Geometry check sheet. Reference: the model listing, model coordinates, mm. Round coordinates to 2 decimals unless told otherwise and drop trailing zeros. Write each loop counter-clockwise with the first axis right and the second up, starting at its lowest first coordinate (ties: lowest second). Pieces come first, ordered by that corner, then holes. Notation, with made-up numbers: M 37,11 L 53,11 A17 cw 53,25 Z; hole C 31,42.5 d4. An arc over 180 degrees is marked long. One line per item, written item: value. Start each with the question number.
1. Section check B-B (y = 2.05). Record the boundary of the cut face in (x, z).
2. Scan lines: probe 1 along X at (y, z) = (1.3, -57.15); probe 2 along X at (y, z) = (1.05, -23.5); probe 3 along X at (y, z) = (2.45, 20). Record each from-to range of solid material in increasing order. Write a range as [from, to].
3. Section check D-D (x = -40). Record the boundary of the cut face in (y, z) (3 decimals), and give its area (3 significant figures).
4. Section check A-A (z = 0). Record the boundary of the cut face in (x, y) (3 decimals).
5. Release check for a two-part mould opening along X. For faces 1 (the flat face through (1, 0, 16)), 2 (the cylindrical face through (0.73, 1.57, 60.45)), 3 (the cylindrical face through (-46.367, 1.565, -60.47)) record: pulls with the +X half, pulls with the -X half, needs draft (parallel to the pull), parting line crosses it, or undercut.
6. Depth check by flat-ended pin: P1, Ø5, axis at x = -45, z = -43, coming from the -Y side; P2, Ø5.5, axis at x = 0, z = 0, coming from the -Y side. Enter the tip coordinate at first touch or a pass-through.
7. Section check C-C (z = 57.15). Record the boundary of the cut face in (x, y) (3 decimals).
from build123d import *

# Parameters (mm, degrees)
SKETCH2_R               = 76.2
BOSS_EXTRUDE1_DEPTH     = 3.175
F_1_4_CLEARANCE_HOLE1_D = 6.7564
F_1_4_CLEARANCE_HOLE2_D = 6.7564


with BuildPart() as part:
    # Sketch2 → Boss-Extrude1 (new body)
    with BuildSketch(Plane(origin=(0, 0, 0), x_dir=(1, 0, 0), z_dir=(0, 1, 0))):
        with Locations(Location((0, 0, 0), (0, 0, 270))):
            Circle(SKETCH2_R)
    extrude(amount=BOSS_EXTRUDE1_DEPTH)

    # 1/4 Clearance Hole1 (through all)
    with Locations(Plane(origin=(0, 3.175, 0), x_dir=(1, 0, 0), z_dir=(0, 1, 0))):
        with Locations((0, 57.15), (0, -57.15)):
            Hole(F_1_4_CLEARANCE_HOLE1_D / 2)

    # 1/4 Clearance Hole2 (through all)
    with Locations(Plane(origin=(0, 3.175, 0), x_dir=(1, 0, 0), z_dir=(0, 1, 0))):
        with Locations((0, 0)):
            Hole(F_1_4_CLEARANCE_HOLE2_D / 2)


solid = part.part
Result sheet:
1. outline: C 0,0 d152.4; hole C 0,-57.15 d6.76; hole C 0,0 d6.76; hole C 0,57.15 d6.76
2. probe 1: x = [-50.4, -3.38], [3.38, 50.4]
2. probe 2: x = [-72.49, 72.49]
2. probe 3: x = [-73.53, 73.53]
3. outline: M 0,-64.857 L 3.175,-64.857 L 3.175,64.857 L 0,64.857 Z
3. area: 412 mm2
4. outline: M -76.2,0 L -3.378,0 L -3.378,3.175 L -76.2,3.175 Z; M 3.378,0 L 76.2,0 L 76.2,3.175 L 3.378,3.175 Z
5. face 1: needs draft
5. face 2: undercut
5. face 3: parting line crosses it
6. P1: stops at y = 0
6. P2: passes through
7. outline: M -50.402,0 L -3.378,0 L -3.378,3.175 L -50.402,3.175 Z; M 3.378,0 L 50.402,0 L 50.402,3.175 L 3.378,3.175 Z
